```python
from build123d import *

# Parameters (mm, degrees)
SKETCH1_R           = 2.5
BOSS_EXTRUDE3_DEPTH = 30
SKETCH4_W           = 40
SKETCH4_H           = 40
BOSS_EXTRUDE5_DEPTH = 5
SKETCH5_W           = 20
SKETCH5_H           = 20
BOSS_EXTRUDE6_DEPTH = 5


with BuildPart() as part:
    # Sketch1 → Boss-Extrude3 (new body)
    with BuildSketch(Plane(origin=(0, 0, 0), x_dir=(1, 0, 0), z_dir=(0, 1, 0))):
        with Locations(Location((10, -10, 0), (0, 0, 270))):  # turned: the seam where the file's is
            Circle(SKETCH1_R)
    extrude(amount=BOSS_EXTRUDE3_DEPTH)

    # Sketch4 → Boss-Extrude5 (add)
    with BuildSketch(Plane(origin=(0, 30, 0), x_dir=(1, 0, 0), z_dir=(0, 1, 0))):
        with Locations((10, -10)):
            Rectangle(SKETCH4_W, SKETCH4_H)
    extrude(amount=BOSS_EXTRUDE5_DEPTH)

    # Sketch5 → Boss-Extrude6 (add)
    with BuildSketch(Plane.XZ):
        with Locations((10, 8.405143714)):
            Rectangle(SKETCH5_W, SKETCH5_H)
    extrude(amount=BOSS_EXTRUDE6_DEPTH)


solid = part.part
```
Here's how the part is built. I have some questions about the finished solid (model axes, mm). A direction names the side the tool comes from. Round coordinates to 2 decimals unless told otherwise and drop trailing zeros. Order: outer loops, then holes, each group sorted by start corner. A loop starts at its lowest first (then second) coordinate and runs counter-clockwise, first axis right, second up. Notation, with made-up numbers: (-36.5, 30) -> (10.5, 30) arc R34 cw to (10.5, 61) -> close; hole circle Ø5 at (15.25, 58.25). An arc over 180 degrees is marked (long way). Use a Markdown table: item, result. Add a question column.
(1) Suppose I cut it at C-C, the plane y = 21. Please give me the cut outline in (x, z), and give its area (3 significant figures).
(2) If we mould it in two halves opening along Y, with no side actions, what happens to faces 1 (the face through (7.56, 14.79, 9.46)), 2 (the face through (20, -2, 8)), 3 (the face through (10, -5, 9))? For each: released by +Y, released by -Y, zero draft, split by the parting line, or undercut.
(3) Suppose I cut it at D-D, the plane x = 10. Please give me the cut outline in (y, z).
(4) For faces 4 (the face through (10, 32, -10)), 5 (the face through (10, -2, -1.595)), 6 (the face through (10, -2, 18.405)), 7 (the face through (0, -2, 8)), 8 (the face through (30, 32, 10)), which set-ups out of +Z, -Z, +X, -X, +Y, -Y let a thin tool reach every point of the face, with its end or its side?
(5) Suppose I cut it at B-B, the plane x = 18. Please give me the cut outline in (y, z), and give its area (3 significant figures).
(6) I need wall thicknesses on line 1 along Y through (x, z) = (13.5, 15.5); line 2 along Y through (x, z) = (26, 19.5); line 3 along Z through (x, y) = (1.5, -1). Which ranges of each line are inside material? Lowest first, please.
(7) Suppose I cut it at A-A, the plane z = 14. Please give me the cut outline in (x, y), and give its area (3 significant figures).
(8) For pin 1 Ø5.5 at (x, y) = (14, -2) entering from +Z; pin 2 Ø2.5 at (y, z) = (-2, 4.5) entering from +X; pin 3 Ø1.5 at (y, z) = (-1.5, 11.5) entering from -X; pin 4 Ø8 at (y, z) = (9, 3) entering from +X, each with a flat end and sliding along its axis, tell me the tip position at first contact or that it passes through.
Verdict:
| question | item | result |
|---|---|---|
| 1 | outline | circle Ø5 at (10, 10) |
| 1 | area | 19.6 mm2 |
| 2 | face 1 | undercut |
| 2 | face 2 | zero draft |
| 2 | face 3 | released by -Y |
| 3 | outline | (-5, -1.59) -> (0, -1.59) -> (0, 7.5) -> (30, 7.5) -> (30, -10) -> (35, -10) -> (35, 30) -> (30, 30) -> (30, 12.5) -> (0, 12.5) -> (0, 18.41) -> (-5, 18.41) -> close |
| 4 | face 4 | -Z, +X, -X, +Y, -Y |
| 4 | face 5 | -Z, +X, -X, -Y |
| 4 | face 6 | +Z, +X, -X, -Y |
| 4 | face 7 | +Z, -Z, -X, -Y |
| 4 | face 8 | +Z, -Z, +X, +Y, -Y |
| 5 | outline | (-5, -1.59) -> (0, -1.59) -> (0, 18.41) -> (-5, 18.41) -> close; (30, -10) -> (35, -10) -> (35, 30) -> (30, 30) -> close |
| 5 | area | 300 mm2 |
| 6 | line 1 | -5 to 0, 30 to 35 |
| 6 | line 2 | 30 to 35 |
| 6 | line 3 | -1.59 to 18.41 |
| 7 | outline | (-10, 30) -> (30, 30) -> (30, 35) -> (-10, 35) -> close; (0, -5) -> (20, -5) -> (20, 0) -> (0, 0) -> close |
| 7 | area | 300 mm2 |
| 8 | pin 1 | z = 18.41 |
| 8 | pin 2 | x = 20 |
| 8 | pin 3 | x = 0 |
| 8 | pin 4 | through |
